Check sheet for the modelled part. Datum: model origin and axes. Units: mm. A direction names the side the tool comes from. Coordinates: 2 decimals unless noted, no trailing zeros. Write each loop counter-clockwise with the first axis right and the second up, starting at its lowest first coordinate (ties: lowest second). Pieces come first, ordered by that corner, then holes. Notation, with made-up numbers: (69, -21.5) -> (128, -21.5) arc R22 ccw to (128, 8.5) -> close; hole circle Ø7 at (-2, 43.5). An arc over 180 degrees is marked (long way). One line per item, written item: value. Start each with the question number.
1) Set-up check for faces 4 (the flat face through (-5, -6, 1.6)), 5 (the flat face through (-24, 23.4, 49)), 6 (the cylindrical face through (-5.56, 24.43, 9.4)), 7 (the flat face through (-21.6, -17, 66)): record each of +Z, -Z, +X, -X, +Y, -Y from which the full face is reachable in a straight line by a thin tool's end or side.
2) Gauge pin test, flat ends, axial feed: P1, Ø14, axis at y = -9, z = 52, coming from the +X side; P2, Ø8, axis at x = -19.5, y = -4.5, coming from the -Z side; P3, Ø3, axis at x = -3, y = -4.5, coming from the +Z side. Record the tip position at first contact, or that the pin passes through.
3) Sectioned sample at C-C on z = 25.5. Enter the section's corners in (x, y), plus the area to 3 significant figures.
4) Sectioned sample at A-A on x = -8.5. Enter the section's corners in (y, z).
5) Scan lines: line 1 along Y through (x, z) = (-25.5, 27); line 2 along X through (y, z) = (-14, 23.5); line 3 along Y through (x, z) = (-7, 8). Record each from-to range of solid material in increasing order. Write a range as [from, to].
6) Sectioned sample at B-B on y = -4. Enter the section's corners in (x, z).
7) Draft check along Y on faces 1 (the cylindrical face through (-29.4, -24.43, 65.12)), 2 (the cylindrical face through (-22.87, -6.12, 6.85)), 3 (the flat face through (-6, 0, 10)). Enter one of: +Y half, -Y half, draft (parallel to the pull), parting line (faces both ways), or undercut.
```python
from build123d import *

# Parameters (mm, degrees)
SKETCH_W    = 50
SKETCH_H    = 10
SKETCH_W_2  = 10.5
SKETCH_H_2  = 6.8
FILLET_R    = 2
FILLET001_R = 2
FILLET002_R = 2
FILLET003_R = 2
FILLET004_R = 1
FILLET005_R = 1


with BuildPart() as part:
    # AdditivePipe: sweep along a path in Sketch001
    with BuildLine(Plane.XZ) as additivepipe_path:
        Line((0, 0), (-10, 0))
        ThreePointArc((-10, 0), (-24.142136, 5.857864), (-30, 20))
        Line((-30, 20), (-30, 110))
    # Sketch → AdditivePipe (sweep)
    with BuildSketch(Plane.YZ):
        with Locations((0, 5)):
            Rectangle(SKETCH_W, SKETCH_H)
        with Locations((-18.15, 5)):
            Rectangle(SKETCH_W_2, SKETCH_H_2, mode=Mode.SUBTRACT)
        with Locations((-6.05, 5)):
            Rectangle(SKETCH_W_2, SKETCH_H_2, mode=Mode.SUBTRACT)
        with Locations((6.05, 5)):
            Rectangle(SKETCH_W_2, SKETCH_H_2, mode=Mode.SUBTRACT)
        with Locations((18.15, 5)):
            Rectangle(SKETCH_W_2, SKETCH_H_2, mode=Mode.SUBTRACT)
    sweep(path=additivepipe_path.line)

    # Fillet
    fillet_edges = [part.edges().sort_by_distance(p)[0] for p in [
        (-20, -25, 65),
        (-17.071068, -25, 12.928932),
        (-5, -25, 10),
        (-20, 25, 65),
        (-17.071068, 25, 12.928932),
        (-5, 25, 10),
    ]]
    fillet(fillet_edges, radius=FILLET_R)

    # Fillet001
    fillet001_edges = [part.edges().sort_by_distance(p)[0] for p in [
        (-5, 25, 0),
        (-24.142136, 25, 5.857864),
        (-30, 25, 65),
        (-30, -25, 65),
        (-24.142136, -25, 5.857864),
        (-5, -25, 0),
    ]]
    fillet(fillet001_edges, radius=FILLET001_R)

    # Fillet002
    fillet002_edges = [part.edges().sort_by_distance(p)[0] for p in [
        (-28.4, -23.4, 65),
        (-21.6, -23.4, 65),
        (-23.010765, -23.4, 6.989235),
        (-18.202439, -23.4, 11.797561),
        (-5, -23.4, 8.4),
        (-5, -23.4, 1.6),
    ]]
    fillet(fillet002_edges, radius=FILLET002_R)

    # Fillet003
    fillet003_edges = [part.edges().sort_by_distance(p)[0] for p in [
        (-28.4, 23.4, 65),
        (-21.6, 23.4, 65),
        (-23.010765, 23.4, 6.989235),
        (-18.202439, 23.4, 11.797561),
        (-5, 23.4, 8.4),
        (-5, 23.4, 1.6),
    ]]
    fillet(fillet003_edges, radius=FILLET003_R)

    # Fillet004
    fillet004_edges = [part.edges().sort_by_distance(p)[0] for p in [
        (0, 0, 10),
        (0, -24.414214, 9.414214),
        (0, -25, 5),
        (0, -24.414214, 0.585786),
        (0, 0, 0),
        (0, 24.414214, 0.585786),
        (0, 25, 5),
        (0, 24.414214, 9.414214),
    ]]
    fillet(fillet004_edges, radius=FILLET004_R)

    # Fillet005
    fillet005_edges = [part.edges().sort_by_distance(p)[0] for p in [
        (-20, 0, 110),
        (-20.585786, -24.414214, 110),
        (-25, -25, 110),
        (-29.414214, -24.414214, 110),
        (-30, 0, 110),
        (-29.414214, 24.414214, 110),
        (-25, 25, 110),
        (-20.585786, 24.414214, 110),
    ]]
    fillet(fillet005_edges, radius=FILLET005_R)


solid = part.part
```
Answers:
1. face 4: +X
1. face 5: none
1. face 6: +Z, +X, +Y
1. face 7: +Z
2. P1: stops at x = -20
2. P2: stops at z = 0.77
2. P3: stops at z = 10
3. outline: (-30, -23) arc R2 ccw to (-28, -25) -> (-22, -25) arc R2 ccw to (-20, -23) -> (-20, 23) arc R2 ccw to (-22, 25) -> (-28, 25) arc R2 ccw to (-30, 23) -> close; hole (-28.4, -21.4) arc R2 ccw to (-26.4, -23.4) -> (-23.6, -23.4) arc R2 ccw to (-21.6, -21.4) -> (-21.6, -12.9) -> (-28.4, -12.9) -> close; hole (-28.4, -11.3) -> (-21.6, -11.3) -> (-21.6, -0.8) -> (-28.4, -0.8) -> close; hole (-28.4, 0.8) -> (-21.6, 0.8) -> (-21.6, 11.3) -> (-28.4, 11.3) -> close; hole (-28.4, 12.9) -> (-21.6, 12.9) -> (-21.6, 21.4) arc R2 ccw to (-23.6, 23.4) -> (-26.4, 23.4) arc R2 ccw to (-28.4, 21.4) -> close
3. area: 214 mm2
4. outline: (-25, 2) arc R2 ccw to (-23, 0) -> (23, 0) arc R2 ccw to (25, 2) -> (25, 8) arc R2 ccw to (23, 10) -> (-23, 10) arc R2 ccw to (-25, 8) -> close; hole (-23.4, 3.6) arc R2 ccw to (-21.4, 1.6) -> (-12.9, 1.6) -> (-12.9, 8.4) -> (-21.4, 8.4) arc R2 ccw to (-23.4, 6.4) -> close; hole (-11.3, 1.6) -> (-0.8, 1.6) -> (-0.8, 8.4) -> (-11.3, 8.4) -> close; hole (0.8, 1.6) -> (11.3, 1.6) -> (11.3, 8.4) -> (0.8, 8.4) -> close; hole (12.9, 1.6) -> (21.4, 1.6) arc R2 ccw to (23.4, 3.6) -> (23.4, 6.4) arc R2 ccw to (21.4, 8.4) -> (12.9, 8.4) -> close
5. line 1: y = [-25, -23.4], [-12.9, -11.3], [-0.8, 0.8], [11.3, 12.9], [23.4, 25]
5. line 2: x = [-30, -28.4], [-21.6, -20]
5. line 3: y = [-25, -22.6], [-12.9, -11.3], [-0.8, 0.8], [11.3, 12.9], [22.6, 25]
6. outline: (-30, 20) arc R20 ccw to (-10, 0) -> (-1, 0) arc R1 ccw to (0, 1) -> (0, 1.6) -> (-10, 1.6) arc R18.4 cw to (-28.4, 20) -> (-28.4, 110) -> (-29, 110) arc R1 ccw to (-30, 109) -> close; (-21.6, 20) arc R11.6 ccw to (-10, 8.4) -> (0, 8.4) -> (0, 9) arc R1 ccw to (-1, 10) -> (-10, 10) arc R10 cw to (-20, 20) -> (-20, 109) arc R1 ccw to (-21, 110) -> (-21.6, 110) -> close
7. face 1: -Y half
7. face 2: undercut
7. face 3: draft
